```python
from build123d import *

# Parameters (mm, degrees)
F0_W      = 31
F0_H      = 18.3
F0_W_2    = 26.2
F0_H_2    = 13.5
F1_DEPTH  = 17.5
F2_W      = 26.2
F2_H      = 13.5
F2_W_2    = 22.2
F2_H_2    = 9.5
F3_DEPTH  = 2
F4_SIZE   = 1.99999
F6_START  = 13
F5_R      = 1.5
F6_DEPTH  = 4.5
F8_DEPTH  = 3
F10_DEPTH = 5
F11_R     = 1.49999
F12_R     = 3


# Not quite as in the source:
# - a fillet or chamfer is up to 0.001 mm smaller than in the source, because OpenCascade refuses the exact size


with BuildPart() as f1:
    # F0 (on Top) → F1 (new body)
    with BuildSketch(Plane.XY):
        Rectangle(F0_W, F0_H)
        Rectangle(F0_W_2, F0_H_2, mode=Mode.SUBTRACT)
    extrude(amount=F1_DEPTH)

    # F2 (on face) → F3 (join)
    with BuildSketch(Plane(origin=(0, 0, 0), x_dir=(1, 0, 0), z_dir=(0, 0, -1))):
        Rectangle(F2_W, F2_H)
        Rectangle(F2_W_2, F2_H_2, mode=Mode.SUBTRACT)
    extrude(amount=-F3_DEPTH)

    # F4 (size 2 in the source; OpenCascade refuses exactly that, so slightly less here)
    f4_edges = [f1.edges().sort_by_distance(p)[0] for p in [
        (0, 4.75, 2),
        (11.1, 0, 2),
        (0, -4.75, 2),
        (-11.1, 0, 2),
    ]]
    chamfer(f4_edges, length=F4_SIZE)

    # F5 (on Top) → F6 (join)
    with BuildSketch(Plane.XY.offset(F6_START)):
        with BuildLine():
            Line((17.1, -4), (21.1, -4))
            ThreePointArc((21.1, -4), (25.1, 0), (21.1, 4))
            Line((21.1, 4), (17.1, 4))
            Line((17.1, 4), (15.5, 4))
            Line((15.5, 4), (15.5, -4))
            Line((15.5, -4), (17.1, -4))
        make_face()
        with Locations((21.1, 0)):
            Circle(F5_R, mode=Mode.SUBTRACT)
        with BuildLine():
            ThreePointArc((-21.1, 4), (-25.1, 0), (-21.1, -4))
            Line((-21.1, -4), (-17.1, -4))
            Line((-17.1, -4), (-15.5, -4))
            Line((-15.5, -4), (-15.5, 4))
            Line((-15.5, 4), (-17.1, 4))
            Line((-17.1, 4), (-21.1, 4))
        make_face()
        with Locations((-21.1, 0)):
            Circle(F5_R, mode=Mode.SUBTRACT)
    extrude(amount=F6_DEPTH)

    # F7 (on face) → F8 (cut)
    with BuildSketch(Plane(origin=(0, 0, 13), x_dir=(1, 0, 0), z_dir=(0, 0, -1))):
        Polygon((22.6877132403, 2.75), (19.5122867597, 2.75), (17.9245735195, 0), (19.5122867597, -2.75), (22.6877132403, -2.75), (24.2754264805, 0), align=None)
        Polygon((-19.5122867597, 2.75), (-22.6877132403, 2.75), (-24.2754264805, 0), (-22.6877132403, -2.75), (-19.5122867597, -2.75), (-17.9245735195, 0), align=None)
    extrude(amount=-F8_DEPTH, mode=Mode.SUBTRACT)

    # F9 (on face) → F10 (cut)
    with BuildSketch(Plane.YZ.offset(15.5)):
        Polygon((0.75, 5.25), (2.5, 5.25), (2.5, 6.75), (-2.5, 6.75), (-2.5, 5.25), (-0.75, 5.25), (-0.75, 0), (0.75, 0), align=None)
    extrude(amount=-F10_DEPTH, mode=Mode.SUBTRACT)

    # F11 (radius 1.5 in the source; OpenCascade refuses exactly that, so slightly less here)
    f11_edges = [f1.edges().sort_by_distance(p)[0] for p in [
        (14.3, -2.5, 5.25),
        (14.3, 2.5, 5.25),
    ]]
    fillet(f11_edges, radius=F11_R)

    # F12
    f12_edges = [f1.edges().sort_by_distance(p)[0] for p in [
        (14.3, -0.75, 5.25),
        (14.3, 0.75, 5.25),
    ]]
    fillet(f12_edges, radius=F12_R)


solid = f1.part
```
Verification items for the finished model (mm, model axes). A direction names the side the tool comes from. Coordinates: 2 decimals unless noted, no trailing zeros. Write each loop counter-clockwise with the first axis right and the second up, starting at its lowest first coordinate (ties: lowest second). Pieces come first, ordered by that corner, then holes. Notation, with made-up numbers: M 59.5,29 L 112.5,29 A36 ccw 112.5,67 Z; hole C 46.5,-15 d10. An arc over 180 degrees is marked long. Answer as a JSON object with one key per item and string values. Group by question number.
(1) Tool access check on faces 4 (the face through (-18, 4, 15)), 5 (the face through (14, -0.75, 1)), 6 (the face through (21, 2.75, 14)). Record the directions out of +Z, -Z, +X, -X, +Y, -Y that give a thin tool (end or side, any length) a straight path to the whole face; none if there is none.
(2) Gauge pin test, flat ends, axial feed: pin 1 (0.9 mm diameter, centred on x = 21.5, z = 14, fed in from +Y); pin 2 (3.5 mm diameter, centred on x = -20.5, z = 15, fed in from -Y); pin 3 (7 mm diameter, centred on y = -2.5, z = 7, fed in from +X). Record the tip position at first contact, or that the pin passes through.
(3) Release check for a two-part mould opening along Y. For faces 1 (the face through (-19.67, 0.45, 16.74)), 2 (the face through (18, -4, 15)), 3 (the face through (2, 7, 17.5)) record: +Y half, -Y half, draft (parallel to the pull), parting line (faces both ways), or undercut.
(4) Cross-section at D-D, the plane z = 1.5. Record the cut outline in (x, y), and give its area (3 significant figures).
(5) Material ranges on line 1 (X direction, y = 0, z = 16.65); line 2 (Y direction, x = -21.1, z = 16.9); line 3 (Y direction, x = 1.5, z = 3.25), recorded low to high.
(6) Cross-section at C-C, the plane z = 8.25. Record the cut outline in (x, y).
(7) Cross-section at B-B, the plane z = 14.5. Record the cut outline in (x, y).
Reply:
{
 "1": {"face 4": "+Z, -Z, -X, +Y", "face 5": "-Z, +X", "face 6": "-Z"},
 "2": {"pin 1": "y = 4", "pin 2": "y = -4", "pin 3": "x = 15.5"},
 "3": {"face 1": "undercut", "face 2": "-Y half", "face 3": "draft"},
 "4": {"outline": "M -15.5,-9.15 L 15.5,-9.15 L 15.5,-0.75 L 12.6,-0.75 L 12.6,-6.25 L -12.6,-6.25 L -12.6,6.25 L 12.6,6.25 L 12.6,0.75 L 15.5,0.75 L 15.5,9.15 L -15.5,9.15 Z", "area": "248 mm²"},
 "5": {"line 1": "-25.1 to -22.6, -19.6 to -13.1, 13.1 to 19.6, 22.6 to 25.1", "line 2": "-4 to -1.5, 1.5 to 4", "line 3": "-9.15 to -6.75, 6.75 to 9.15"},
 "6": {"outline": "M -15.5,-9.15 L 15.5,-9.15 L 15.5,9.15 L -15.5,9.15 Z; hole M -13.1,-6.75 L 13.1,-6.75 L 13.1,6.75 L -13.1,6.75 Z"},
 "7": {"outline": "M -21.1,-4 L -15.5,-4 L -15.5,-9.15 L 15.5,-9.15 L 15.5,-4 L 21.1,-4 A4 ccw 21.1,4 L 15.5,4 L 15.5,9.15 L -15.5,9.15 L -15.5,4 L -21.1,4 A4 ccw Z; hole M -24.28,0 L -22.69,-2.75 L -19.51,-2.75 L -17.92,0 L -19.51,2.75 L -22.69,2.75 Z; hole M -13.1,-6.75 L 13.1,-6.75 L 13.1,6.75 L -13.1,6.75 Z; hole M 17.92,0 L 19.51,-2.75 L 22.69,-2.75 L 24.28,0 L 22.69,2.75 L 19.51,2.75 Z"}
}
